Study the drawing (mm; zero at the part's minimum x, y, z) and answer. Round coordinates to 2 decimals unless told otherwise and drop trailing zeros. Write each loop counter-clockwise with the first axis right and the second up, starting at its lowest first coordinate (ties: lowest second). Pieces come first, ordered by that corner, then holes. Notation, with made-up numbers: (68.5, 75.25) -> (100.5, 75.25) arc R9 cw to (100.5, 88.25) -> close; hole circle Ø8 at (-4.75, 7.5). An arc over 180 degrees is marked (long way). One line per question, with ' | ' between items. Start each with the question number.
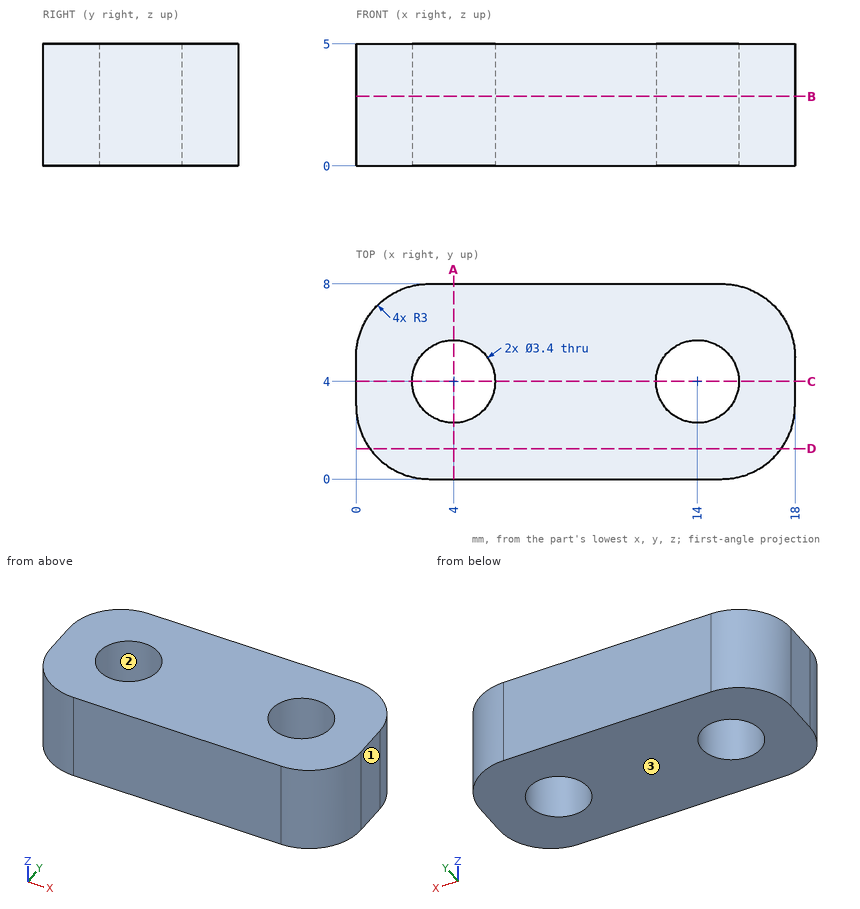
(1) The mould has two halves that part along X. Classify the marked faces 1, 2 and 3: +X half, -X half, draft (parallel to the pull), parting line (faces both ways), or undercut.
(2) Consider L1, parallel to X at y = 4.5, z = 0.5; L2, parallel to X at y = 3.25, z = 3.55; L3, parallel to Y at x = 14, z = 3.65. Determine where each line is inside the solid, lowest interval first.
(3) A cutting plane is placed at C-C, the plane y = 4. Determine the outline of the cut face in (x, z), then the cut area to 3 significant figures.
(4) A cutting plane is placed at D-D, the plane y = 1.25. Determine the outline of the cut face in (x, z), then the cut area to 3 significant figures.
(5) A cutting plane is placed at B-B, the plane z = 2.85. Determine the outline of the cut face in (x, y), then the cut area to 3 significant figures.
(6) Given pin 1 Ø2.5 at (x, y) = (14, 4) entering from -Z; pin 2 Ø1 at (x, z) = (2, 4.5) entering from +Y, each flat-ended and moving along its own axis, determine where each tip first touches the part or whether it passes through.
(7) A cutting plane is placed at A-A, the plane x = 4. Determine the outline of the cut face in (y, z), then the cut area to 3 significant figures.
Returned:
1) face 1: +X half | face 2: undercut | face 3: draft
2) L1: 0 to 2.38, 5.62 to 12.38, 15.62 to 18 | L2: 0 to 2.47, 5.53 to 12.47, 15.53 to 18 | L3: 0 to 2.3, 5.7 to 8
3) outline: (0, 0) -> (2.3, 0) -> (2.3, 5) -> (0, 5) -> close; (5.7, 0) -> (12.3, 0) -> (12.3, 5) -> (5.7, 5) -> close; (15.7, 0) -> (18, 0) -> (18, 5) -> (15.7, 5) -> close | area: 56.0 mm2
4) outline: (0.56, 0) -> (17.44, 0) -> (17.44, 5) -> (0.56, 5) -> close | area: 84.4 mm2
5) outline: (0, 3) arc R3 ccw to (3, 0) -> (15, 0) arc R3 ccw to (18, 3) -> (18, 5) arc R3 ccw to (15, 8) -> (3, 8) arc R3 ccw to (0, 5) -> close; hole circle Ø3.4 at (4, 4); hole circle Ø3.4 at (14, 4) | area: 118 mm2
6) pin 1: through | pin 2: y = 7.96
7) outline: (0, 0) -> (2.3, 0) -> (2.3, 5) -> (0, 5) -> close; (5.7, 0) -> (8, 0) -> (8, 5) -> (5.7, 5) -> close | area: 23.0 mm2
